```python
from build123d import *

# Parameters (mm, degrees)
F0_W     = 300
F0_H     = 200
F0_R     = 15.75
F0_R_2   = 8.75
F1_DEPTH = 40
F2_DEPTH = 20
F3_R     = 50
F4_DEPTH = 40
F5_D     = 15.5
F7_DEPTH = 25
F8_SIZE  = 5


with BuildPart() as f1:
    # F0 (on Top) → F1 (new body)
    with BuildSketch(Plane.XY):
        Rectangle(F0_W, F0_H)
        with Locations((-10, -60)):
            Circle(F0_R, mode=Mode.SUBTRACT)
        with Locations((110, -60)):
            Circle(F0_R, mode=Mode.SUBTRACT)
        with Locations((-10, 60)):
            Circle(F0_R, mode=Mode.SUBTRACT)
        with Locations((110, 60)):
            Circle(F0_R, mode=Mode.SUBTRACT)
        with Locations((-10, 60)):
            Circle(F0_R)
        with Locations((-10, 60)):
            Circle(F0_R_2, mode=Mode.SUBTRACT)
        with Locations((110, 60)):
            Circle(F0_R)
        with Locations((110, 60)):
            Circle(F0_R_2, mode=Mode.SUBTRACT)
        with Locations((-10, -60)):
            Circle(F0_R)
        with Locations((-10, -60)):
            Circle(F0_R_2, mode=Mode.SUBTRACT)
        with Locations((110, -60)):
            Circle(F0_R)
        with Locations((110, -60)):
            Circle(F0_R_2, mode=Mode.SUBTRACT)
    extrude(amount=-F1_DEPTH)

    # F0 (on Top) → F2 (cut)
    with BuildSketch(Plane.XY):
        with Locations((-10, 60)):
            Circle(F0_R)
        with Locations((-10, 60)):
            Circle(F0_R_2, mode=Mode.SUBTRACT)
        with Locations((110, 60)):
            Circle(F0_R)
        with Locations((110, 60)):
            Circle(F0_R_2, mode=Mode.SUBTRACT)
        with Locations((110, -60)):
            Circle(F0_R)
        with Locations((110, -60)):
            Circle(F0_R_2, mode=Mode.SUBTRACT)
        with Locations((-10, -60)):
            Circle(F0_R)
        with Locations((-10, -60)):
            Circle(F0_R_2, mode=Mode.SUBTRACT)
    extrude(amount=-F2_DEPTH, mode=Mode.SUBTRACT)

    # F3 (on face) → F4 (join)
    with BuildSketch(Plane(origin=(-150, 0, 0), x_dir=(0, -1, 0), z_dir=(-1, 0, 0))):
        with BuildLine():
            Line((-100, 160), (-100, -40))
            Line((-100, -40), (100, -40))
            Line((100, -40), (100, 160))
            ThreePointArc((100, 160), (0, 60), (-100, 160))
        make_face()
        with BuildLine():
            ThreePointArc((100, 160), (0, 260), (-100, 160))
            ThreePointArc((-100, 160), (0, 60), (100, 160))
        make_face()
        with Locations((0, 160)):
            Circle(F3_R, mode=Mode.SUBTRACT)
    extrude(amount=F4_DEPTH)

    # F5 (through all)
    with Locations(Plane(origin=(-150, 0, 0), x_dir=(0, -1, 0), z_dir=(1, 0, 0))):
        with Locations((-72, -160), (0, -232), (72, -160), (0, -88)):
            Hole(F5_D / 2)

    # F6 (on Front) → F7 (join, symmetric)
    with BuildSketch(Plane.XZ):
        Polygon((-150, 60), (-150, 0), (-90, 0), align=None)
    extrude(amount=F7_DEPTH, both=True)

    # F8
    f8_edges = [f1.edges().sort_by_distance(p)[0] for p in [
        (150, -100, -20),
        (150, 100, -20),
        (-150, 50, 160),
    ]]
    chamfer(f8_edges, length=F8_SIZE)


solid = f1.part
```
Verification items for the finished model (mm, model axes). A direction names the side the tool comes from. Round coordinates to 2 decimals unless told otherwise and drop trailing zeros. Order: outer loops, then holes, each group sorted by start corner. A loop starts at its lowest first (then second) coordinate and runs counter-clockwise, first axis right, second up.
1) Draft check along Z on faces 1 (the flat face through (-134, 25, 17)), 2 (the cylindrical face through (-172.26, 10.84, 111.19)), 3 (the flat face through (117, -67, -20)). Enter one of: +Z half, -Z half, draft (parallel to the pull), parting line (faces both ways), or undercut.
Geometry says:
face 1: draft
face 2: undercut
face 3: +Z half
2) Depth check by flat-ended pin: pin 1 (9.5 mm diameter, centred on y = -72, z = 160, fed in from +X); pin 2 (18 mm diameter, centred on x = -116, z = 16.5, fed in from -Y); pin 3 (1 mm diameter, centred on y = -26, z = 69.5, fed in from +X); pin 4 (19 mm diameter, centred on x = 110, y = 60, fed in from +Z). Enter the tip coordinate at first touch or a pass-through.
Geometry says:
pin 1: passes through
pin 2: stops at y = -25
pin 3: stops at x = -150
pin 4: stops at z = -20
3) Tool access check on faces 4 (the flat face through (-134, -25, 17)), 5 (the cylindrical face through (-170.28, 65.85, 164.716)), 6 (the flat face through (-3, 53, -20)). Record the directions out of +Z, -Z, +X, -X, +Y, -Y that give a thin tool (end or side, any length) a straight path to the whole face; none if there is none.
Geometry says:
face 4: +Z, +X, -Y
face 5: +X, -X
face 6: +Z
4) Material ranges on line 1 (Z direction, x = -167, y = 0); line 2 (Z direction, x = -69, y = 79.5); line 3 (X direction, y = 60, z = 88), recorded low to high.
Geometry says:
line 1: z = -40 to 80.25, 95.75 to 110, 210 to 224.25, 239.75 to 260
line 2: z = -40 to 0
line 3: x = -190 to -150
5) Cross-section at B-B, the plane z = 88. Record the cut outline in (x, y).
Geometry says:
outline: (-190, -100) - (-150, -100) - (-150, -7.75) - (-190, -7.75) - close; (-190, 7.75) - (-150, 7.75) - (-150, 100) - (-190, 100) - close
6) Cross-section at C-C, the plane y = 0. Record the cut outline in (x, z).
Geometry says:
outline: (-190, -40) - (150, -40) - (150, 0) - (-90, 0) - (-150, 60) - (-150, 80.25) - (-190, 80.25) - close; (-190, 95.75) - (-150, 95.75) - (-150, 105) - (-155, 110) - (-190, 110) - close; (-190, 210) - (-155, 210) - (-150, 215) - (-150, 224.25) - (-190, 224.25) - close; (-190, 239.75) - (-150, 239.75) - (-150, 260) - (-190, 260) - close
7) Cross-section at D-D, the plane x = -48.5. Record the cut outline in (y, z).
Geometry says:
outline: (-100, -40) - (100, -40) - (100, 0) - (-100, 0) - close
8) Cross-section at A-A, the plane y = -60. Record the cut outline in (x, z).
Geometry says:
outline: (-190, -40) - (-18.75, -40) - (-18.75, -20) - (-25.75, -20) - (-25.75, 0) - (-150, 0) - (-150, 240) - (-190, 240) - close; (-1.25, -40) - (101.25, -40) - (101.25, -20) - (94.25, -20) - (94.25, 0) - (5.75, 0) - (5.75, -20) - (-1.25, -20) - close; (118.75, -40) - (150, -40) - (150, 0) - (125.75, 0) - (125.75, -20) - (118.75, -20) - close
